Part model, mm, in its own coordinate system. A direction names the side the tool comes from. Round coordinates to 2 decimals unless told otherwise and drop trailing zeros. Loops run counter-clockwise (first coordinate to the right, second up) from the corner with the lowest first, then second, coordinate; pieces in that order, holes last. Notation, with made-up numbers: (-15, 53) -> (33, 53) arc R14 ccw to (33, 78) -> close; hole circle Ø9 at (-25, 17.25). An arc over 180 degrees is marked (long way). Answer as CSV lines item,"result".
from build123d import *

# Parameters (mm, degrees)
F1_DEPTH = 6.35


with BuildPart() as f1:
    # F0 (on Front) → F1 (new body)
    with BuildSketch(Plane.XZ):
        with BuildLine():
            ThreePointArc((0, 72.4705681205), (-31.6151754834, 51.0205932538), (-58.2285185052, 23.6098158874))
            ThreePointArc((-58.2285185052, 23.6098158874), (-39.747753506, 29.3045872421), (-22.6139344783, 20.3379077418))
            Line((-22.6139344783, 20.3379077418), (-3.1564056231, 36.6647130278))
            ThreePointArc((-3.1564056231, 36.6647130278), (-9.0007564313, 55.2219634474), (0, 72.4705681205))
        make_face()
        with BuildLine():
            Line((-3.1564056231, 36.6647130278), (-22.6139344783, 20.3379077418))
            ThreePointArc((-22.6139344783, 20.3379077418), (-18.2032707655, 12.6984140962), (-16.6714633335, 4.0111024557))
            Line((-16.6714633335, 4.0111024557), (8.7285366665, 4.0111024557))
            ThreePointArc((8.7285366665, 4.0111024557), (8.7325019345, 4.4599007306), (8.7443965005, 4.908558879))
            ThreePointArc((8.7443965005, 4.908558879), (6.1125631722, 21.5486538709), (-2.5673824162, 35.9874160266))
            ThreePointArc((-2.5673824162, 35.9874160266), (-2.8648860812, 36.3234624284), (-3.1564056231, 36.6647130278))
        make_face()
        with BuildLine():
            ThreePointArc((-16.6714633335, 4.0111024557), (-21.7868505138, -11.2759666798), (-35.0726037079, -20.4056123917))
            ThreePointArc((-35.0726037079, -20.4056123917), (-3.9714633335, -16.0361449079), (27.129677041, -20.4056123917))
            ThreePointArc((27.129677041, -20.4056123917), (13.8439238468, -11.2759666798), (8.7285366665, 4.0111024557))
            Line((8.7285366665, 4.0111024557), (-16.6714633335, 4.0111024557))
        make_face()
        with BuildLine():
            ThreePointArc((58.9453417467, -1.4005687843), (56.1752899305, 39.7699962571), (31.833343639, 73.0890338128))
            ThreePointArc((31.833343639, 73.0890338128), (39.10110567, 64.1861956577), (41.7011232322, 52.9915183138))
            ThreePointArc((41.7011232322, 52.9915183138), (41.3188749847, 48.6015186275), (40.18363526, 44.3436504125))
            ThreePointArc((40.18363526, 44.3436504125), (44.2593671036, 35.4329550343), (46.8648599559, 25.9871364261))
            ThreePointArc((46.8648599559, 25.9871364261), (56.1360650551, 16.6929278064), (59.5285366665, 4.0111024557))
            ThreePointArc((59.5285366665, 4.0111024557), (59.382317067, 1.2896000248), (58.9453417467, -1.4005687843))
        make_face()
        with BuildLine():
            ThreePointArc((31.833343639, 73.0890338128), (15.8077391608, 78.3867259751), (0, 72.4705681205))
            ThreePointArc((0, 72.4705681205), (-9.0007564313, 55.2219634474), (-3.1564056231, 36.6647130278))
            Line((-3.1564056231, 36.6647130278), (6.2123223295, 44.5260091974))
            ThreePointArc((6.2123223295, 44.5260091974), (5.5055073041, 46.0788928649), (4.789482931, 47.627551724))
            ThreePointArc((4.789482931, 47.627551724), (8.3636814796, 62.9054992713), (24.0534690987, 63.0508986907))
            ThreePointArc((24.0534690987, 63.0508986907), (33.0695475347, 54.5172622309), (40.18363526, 44.3436504125))
            ThreePointArc((40.18363526, 44.3436504125), (41.3188749847, 48.6015186275), (41.7011232322, 52.9915183138))
            ThreePointArc((41.7011232322, 52.9915183138), (39.10110567, 64.1861956577), (31.833343639, 73.0890338128))
        make_face()
        with BuildLine():
            ThreePointArc((8.7285366665, 4.0111024557), (13.8439238468, -11.2759666798), (27.129677041, -20.4056123917))
            ThreePointArc((27.129677041, -20.4056123917), (47.1541927224, -17.794683114), (58.9453417467, -1.4005687843))
            ThreePointArc((58.9453417467, -1.4005687843), (59.382317067, 1.2896000248), (59.5285366665, 4.0111024557))
            ThreePointArc((59.5285366665, 4.0111024557), (56.1360650551, 16.6929278064), (46.8648599559, 25.9871364261))
            ThreePointArc((46.8648599559, 25.9871364261), (47.9546242088, 13.6208501821), (46.533223206, 1.2882818858))
            ThreePointArc((46.533223206, 1.2882818858), (34.4206876415, -8.6855367771), (21.8622173199, 0.7205995022))
            ThreePointArc((21.8622173199, 0.7205995022), (21.4152650858, 2.3671926108), (20.9585424275, 4.0111024557))
            Line((20.9585424275, 4.0111024557), (8.7285366665, 4.0111024557))
        make_face()
        with BuildLine():
            ThreePointArc((8.7443965005, 4.908558879), (8.7325019345, 4.4599007306), (8.7285366665, 4.0111024557))
            Line((8.7285366665, 4.0111024557), (20.9585424275, 4.0111024557))
            ThreePointArc((20.9585424275, 4.0111024557), (18.3704105721, 12.6927036587), (15.509855789, 21.2883916639))
            ThreePointArc((15.509855789, 21.2883916639), (10.6522338174, 13.7076587794), (8.7443965005, 4.908558879))
        make_face()
        with BuildLine():
            Line((6.2123223295, 44.5260091974), (-3.1564056231, 36.6647130278))
            ThreePointArc((-3.1564056231, 36.6647130278), (-2.8648860812, 36.3234624284), (-2.5673824162, 35.9874160266))
            ThreePointArc((-2.5673824162, 35.9874160266), (4.5500581511, 30.4732486321), (13.1440136398, 27.788489547))
            ThreePointArc((13.1440136398, 27.788489547), (9.8101239891, 36.2118977495), (6.2123223295, 44.5260091974))
        make_face()
        with BuildLine():
            ThreePointArc((13.1440136398, 27.788489547), (4.5500581511, 30.4732486321), (-2.5673824162, 35.9874160266))
            ThreePointArc((-2.5673824162, 35.9874160266), (6.1125631722, 21.5486538709), (8.7443965005, 4.908558879))
            ThreePointArc((8.7443965005, 4.908558879), (10.6522338174, 13.7076587794), (15.509855789, 21.2883916639))
            ThreePointArc((15.509855789, 21.2883916639), (14.3464977034, 24.5455609512), (13.1440136398, 27.788489547))
        make_face()
        with BuildLine():
            ThreePointArc((-22.6139344783, 20.3379077418), (-39.747753506, 29.3045872421), (-58.2285185052, 23.6098158874))
            ThreePointArc((-58.2285185052, 23.6098158874), (-64.5505117579, -7.8148174635), (-35.0726037079, -20.4056123917))
            ThreePointArc((-35.0726037079, -20.4056123917), (-21.7868505138, -11.2759666798), (-16.6714633335, 4.0111024557))
            Line((-16.6714633335, 4.0111024557), (-29.3714633335, 4.0111024557))
            ThreePointArc((-29.3714633335, 4.0111024557), (-54.0055596175, -0.3325533645), (-32.3426989059, 12.1745050987))
            Line((-32.3426989059, 12.1745050987), (-22.6139344783, 20.3379077418))
        make_face()
        with BuildLine():
            ThreePointArc((-16.6714633335, 4.0111024557), (-18.2032707655, 12.6984140962), (-22.6139344783, 20.3379077418))
            Line((-22.6139344783, 20.3379077418), (-32.3426989059, 12.1745050987))
            ThreePointArc((-32.3426989059, 12.1745050987), (-30.1373670495, 8.354758276), (-29.3714633335, 4.0111024557))
            Line((-29.3714633335, 4.0111024557), (-16.6714633335, 4.0111024557))
        make_face()
    extrude(amount=F1_DEPTH)


solid = f1.part
Q1. Saw through at A-A, the plane y = -2. Write the cut outline in (x, z).
Geometry results:
outline,"(-58.23, 23.61) arc R25.4 ccw to (-35.07, -20.41) arc R112.87 cw to (27.13, -20.41) arc R25.4 ccw to (58.95, -1.4) arc R74.17 ccw to (31.83, 73.09) arc R25.4 ccw to (0, 72.47) arc R187.58 ccw to start; hole circle Ø25.4 at (-42.07, 4.01); hole (4.79, 47.63) arc R287.31 cw to (20.96, 4.01) arc R287.31 cw to (21.86, 0.72) arc R12.7 ccw to (46.53, 1.29) arc R61.37 ccw to (24.05, 63.05) arc R12.7 ccw to start"
Q2. Drill centre lines: line 1 along X through (y, z) = (-3.25, 10.5); line 2 along X through (y, z) = (-4, 15); line 3 along Z through (x, y) = (-39.5, -1.5). Where is each one in solid material? Low to high.
Geometry results:
line 1,"-66.63 to -52.99, -31.15 to 19.05, 47.83 to 60.55"
line 2,"-64.97 to -48.44, -35.7 to 17.63, 47.96 to 60.65"
line 3,"-21.26 to -8.43, 16.45 to 44.02"
Q3. Saw through at C-C, the plane z = 51.5. Write the cut outline in (x, y), then the cut area to 3 significant figures.
Geometry results:
outline,"(-31.04, -6.35) -> (3.69, -6.35) -> (3.69, 0) -> (-31.04, 0) -> close; (35.51, -6.35) -> (50.7, -6.35) -> (50.7, 0) -> (35.51, 0) -> close"
area,"317 mm2"
Q4. Which spindle directions (+Z, -Z, +X, -X, +Y, -Y) get a long thin tool onto all of the face, cutting with end or side? Do faces 4 (the face through (-4, -6.35, 18)), 5 (the face through (34.657, -3.131, -8.678)). Say none if no direction does.
Geometry results:
face 4,"+Z, -Z, +X, -X, -Y"
face 5,"+Y, -Y"
Q5. Saw through at D-D, the plane z = 68. Write the cut outline in (x, y), then the cut area to 3 significant figures.
Geometry results:
outline,"(-7.84, -6.35) -> (37.75, -6.35) -> (37.75, 0) -> (-7.84, 0) -> close"
area,"289 mm2"
Q6. Saw through at B-B, the plane x = -45.5. Write the cut outline in (y, z), then the cut area to 3 significant figures.
Geometry results:
outline,"(-6.35, -21.16) -> (0, -21.16) -> (0, -8.22) -> (-6.35, -8.22) -> close; (-6.35, 16.24) -> (0, 16.24) -> (0, 38.12) -> (-6.35, 38.12) -> close"
area,"221 mm2"
Q7. Two-plate mould, pull along X, no slides. Class faces 1 (the face through (-31.204, -3.131, 51.364)), 2 (the face through (-4.413, -3.131, -16.037)), 3 (the face through (-4, 0, 18)): pulls with the +X half, pulls with the -X half, needs draft (parallel to the pull), parting line crosses it, or undercut.
Geometry results:
face 1,"pulls with the -X half"
face 2,"undercut"
face 3,"needs draft"
Q8. Drop a flat-ended pin along its axis: P1, Ø1, axis at x = 24, y = -1.5, coming from the -Z side. Give the stop position or say it passes through.
Geometry results:
P1,"z = -19.69"
